Print and shaded views of the part. All mm, measured from the part's lowest x, y and z. Give positions to 0.01 mm unless a question says otherwise; leave off trailing zeros. Loops run counter-clockwise (first coordinate to the right, second up) from the corner with the lowest first, then second, coordinate; pieces in that order, holes last. Notation, with made-up numbers: M 86,82 L 98,82 A16 ccw 98,104 Z; hole C 40,76.5 d3. An arc over 180 degrees is marked long. Answer in a Markdown table with one row per item.
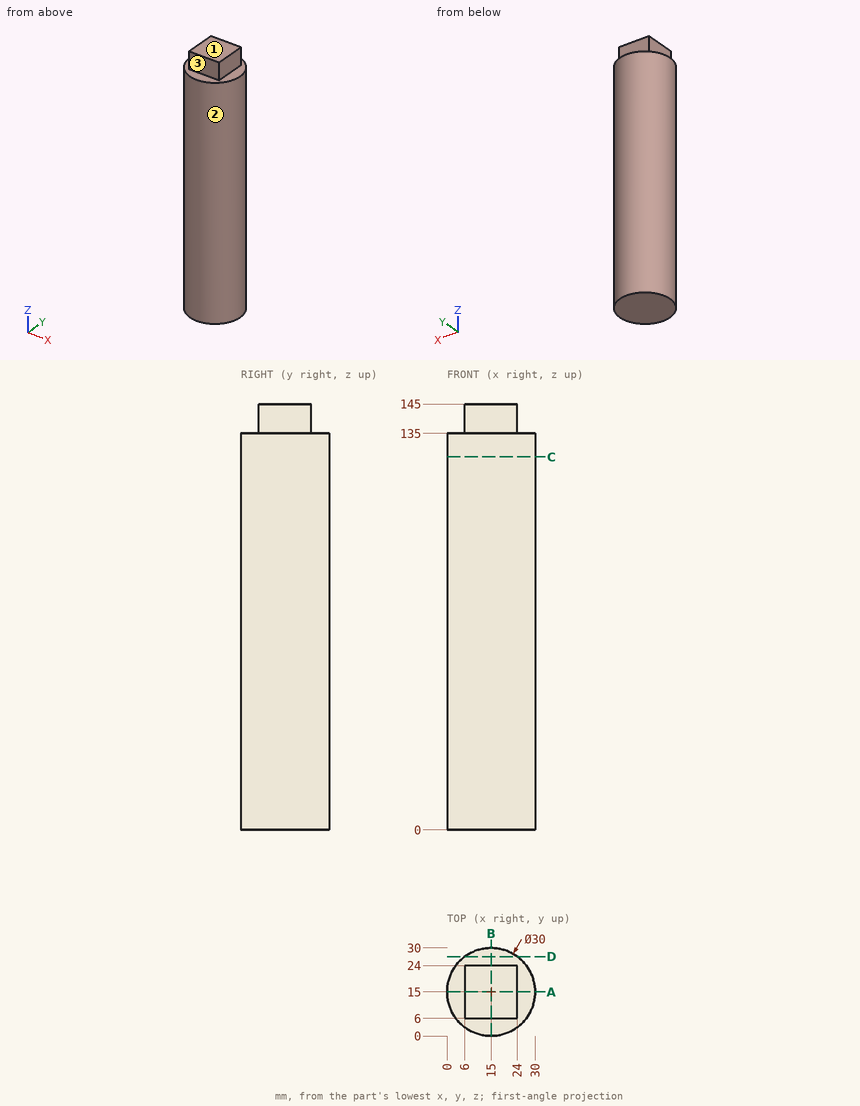
(1) Mould opens along Y. For the marked faces 1, 2 and 3 say: pulls with the +Y half, pulls with the -Y half, needs draft (parallel to the pull), parting line crosses it, or undercut.
Established:
| item | result |
|---|---|
| face 1 | needs draft |
| face 2 | parting line crosses it |
| face 3 | pulls with the -Y half |
(2) Saw through at A-A, the plane y = 15. Give the cut face in (x, z).
Established:
| item | result |
|---|---|
| outline | M 0,0 L 30,0 L 30,135 L 24,135 L 24,145 L 6,145 L 6,135 L 0,135 Z |
(3) Saw through at D-D, the plane y = 27. Give the cut face in (x, z), and give its area (3 significant figures).
Established:
| item | result |
|---|---|
| outline | M 6,0 L 24,0 L 24,135 L 6,135 Z |
| area | 2,430 mm2 |
(4) Wall check: L1, parallel to Z at x = 27, y = 17.75; L2, parallel to Y at x = 15.25, z = 21.5; L3, parallel to X at y = 8.5, z = 86. Give the ranges that are in metal, low to high.
Established:
| item | result |
|---|---|
| L1 | z = 0 to 135 |
| L2 | y = 0 to 30 |
| L3 | x = 1.48 to 28.52 |
(5) Flat gauge pins, fed straight in: P1, Ø3, axis at x = 15, z = 140.5, coming from the -Y side; P2, Ø8, axis at y = 9.5, z = 111.5, coming from the -X side; P3, Ø1, axis at x = 13, z = 59.5, coming from the -Y side. Where does each tip first touch, or does it go through?
Established:
| item | result |
|---|---|
| P1 | stops at y = 6 |
| P2 | stops at x = 0.08 |
| P3 | stops at y = 0.08 |
(6) Saw through at C-C, the plane z = 127. Give the cut face in (x, y), and give its area (3 significant figures).
Established:
| item | result |
|---|---|
| outline | C 15,15 d30 |
| area | 707 mm2 |
